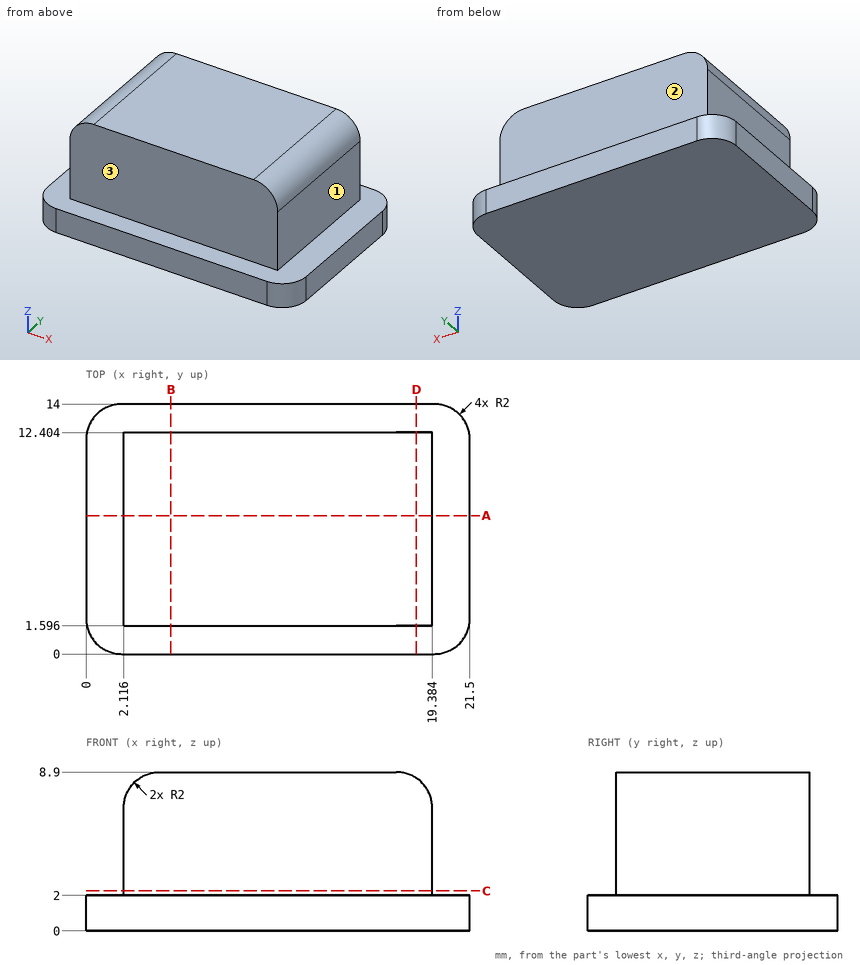
Job drawing, mm, ordinate dimensions from the low corner. One solid piece. A direction names the side the tool comes from. Coordinates: 2 decimals unless noted, no trailing zeros. Write each loop counter-clockwise with the first axis right and the second up, starting at its lowest first coordinate (ties: lowest second). Pieces come first, ordered by that corner, then holes. Notation, with made-up numbers: M 2.25,49.5 L 31.25,49.5 A16 ccw 31.25,68.5 Z; hole C -9,4 d3. An arc over 180 degrees is marked long. Answer as a JSON object with one key per item and string values. Group by question number.
1) Saw through at C-C (z = 2.25). Write the cut outline in (x, y) (1 decimal), plus the area to 3 significant figures.
2) Tool access for the marked faces 1, 2 and 3: list every direction of +Z, -Z, +X, -X, +Y, -Y with a clear straight run to the whole face (end or side of a thin tool).
3) Saw through at D-D (x = 18.5). Write the cut outline in (y, z) (1 decimal), plus the area to 3 significant figures.
4) Saw through at A-A (y = 7.75). Write the cut outline in (x, z).
5) Pin check, flat tips, straight feed: pin 1 Ø1.5 at (x, z) = (12, 6) entering from -Y; pin 2 Ø4 at (y, z) = (6, 5.5) entering from -X; pin 3 Ø2.5 at (y, z) = (5, 5) entering from +X. Stop position of each tip, or through.
6) Saw through at B-B (x = 4.75). Write the cut outline in (y, z) (1 decimal).
7) Wall check: line 1 (X direction, y = 10.75, z = 3.25); line 2 (Z direction, x = 1, y = 13.25); line 3 (Y direction, x = 3, z = 6.5) (1 decimal). Give the ranges that are in metal, low to high. Write a range as from..to.
Values follow:
{
 "1": {"outline": "M 2.1,1.6 L 19.4,1.6 L 19.4,12.4 L 2.1,12.4 Z", "area": "187 mm2"},
 "2": {"face 1": "+Z, +X, +Y, -Y", "face 2": "+Z, +X, -X, +Y", "face 3": "+Z, +X, -X, -Y"},
 "3": {"outline": "M 0,0 L 14,0 L 14,2 L 12.4,2 L 12.4,8.6 L 1.6,8.6 L 1.6,2 L 0,2 Z", "area": "98.9 mm2"},
 "4": {"outline": "M 0,0 L 21.5,0 L 21.5,2 L 19.38,2 L 19.38,6.9 A2 ccw 17.38,8.9 L 4.12,8.9 A2 ccw 2.12,6.9 L 2.12,2 L 0,2 Z"},
 "5": {"pin 1": "stops at y = 1.6", "pin 2": "stops at x = 2.12", "pin 3": "stops at x = 19.38"},
 "6": {"outline": "M 0,0 L 14,0 L 14,2 L 12.4,2 L 12.4,8.9 L 1.6,8.9 L 1.6,2 L 0,2 Z"},
 "7": {"line 1": "x = 2.12..19.38", "line 2": "z = 0..2", "line 3": "y = 1.6..12.4"}
}
